Build history of the part. All positions in model axes, mm. Face numbers are marked on the shaded views. Round coordinates to 2 decimals unless told otherwise and drop trailing zeros. Loops run counter-clockwise (first coordinate to the right, second up) from the corner with the lowest first, then second, coordinate; pieces in that order, holes last. Notation, with made-up numbers: (55, 9.5) - (96, 9.5) arc R16 cw to (96, 34.5) - close; hole circle Ø2 at (1.5, 42.5). An arc over 180 degrees is marked (long way). Use a Markdown table: item, result.
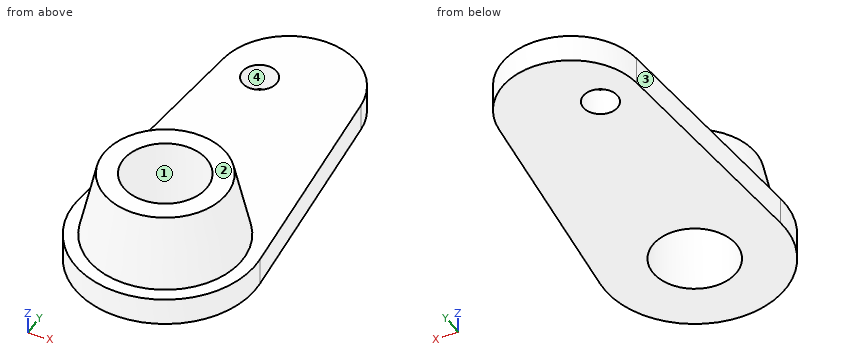
from build123d import *

# Parameters (mm, degrees)
F1_DEPTH = 12.7
F5_D     = 38.1
F7_D     = 15.748


with BuildPart() as f1:
    # F0 (on Top) → F1 (new body)
    with BuildSketch(Plane.XY):
        with BuildLine():
            Line((-31.362119, 109.072947), (-41.099551, 3.801645))
            ThreePointArc((-41.099551, 3.801645), (0, -41.275), (41.099551, 3.801645))
            Line((41.099551, 3.801645), (31.362119, 109.072947))
            ThreePointArc((31.362119, 109.072947), (0, 137.668), (-31.362119, 109.072947))
        make_face()
    extrude(amount=F1_DEPTH)

    # F2 (on Right) → F3 (revolve)
    with BuildSketch(Plane.YZ):
        Polygon((-27.94, 44.45), (-35.052, 12.7), (0, 12.7), (0, 44.45), align=None)
    revolve(axis=Axis((0, 0, 28.575), (0, 0, -1)))

    # F5 (through all)
    with Locations(Plane.XY.offset(44.45)):
        with Locations((0, 0)):
            Hole(F5_D / 2)

    # F7 (through all)
    with Locations(Plane.XY.offset(12.7)):
        with Locations((-12.939112, 105.38061)):
            Hole(F7_D / 2)


solid = f1.part
Q1. Probe line 1 (Y direction, x = -13.5, z = 9.5); line 2 (Z direction, x = 33, y = 58.5); line 3 (Y direction, x = 0, z = 30). List the from-to ranges inside material, lowest first.
Results found:
| item | result |
|---|---|
| line 1 | y = -39 to -13.44, 13.44 to 97.53, 113.23 to 134.63 |
| line 2 | z = 0 to 12.7 |
| line 3 | y = -31.18 to -19.05, 19.05 to 31.18 |
Q2. Cut at C-C, the plane z = 3. List the corners of the cut face in (x, y) (3 decimals).
Results found:
| item | result |
|---|---|
| outline | (-41.1, 3.802) arc R41.275 ccw (long way) to (41.1, 3.802) - (31.362, 109.073) arc R31.496 ccw to (-31.362, 109.073) - close; hole circle Ø15.748 at (-12.939, 105.381); hole circle Ø38.1 at (0, 0) |
Q3. Cut at D-D, the plane z = 37. List the corners of the cut face in (x, y), plus the area to 3 significant figures.
Results found:
| item | result |
|---|---|
| outline | circle Ø59.22 at (0, 0); hole circle Ø38.1 at (0, 0) |
| area | 1,610 mm2 |
Q4. Drop flat-ended pins along their axis: pin 1 (10 mm diameter, centred on x = -26.5, z = 5.5, fed in from -Y); pin 2 (2 mm diameter, centred on x = 11, z = 24, fed in from +Y); pin 3 (1.5 mm diameter, centred on x = 27, z = 38, fed in from +Y). Give the stop position or say it passes through.
Results found:
| item | result |
|---|---|
| pin 1 | stops at y = -35.23 |
| pin 2 | stops at y = 31.02 |
| pin 3 | stops at y = 13.25 |
Q5. Pull direction Y, two halves, no side cores. Call the marked faces 1, 2, 3 and 4: pulls with the +Y half, pulls with the -Y half, needs draft (parallel to the pull), parting line crosses it, or undercut.
Results found:
| item | result |
|---|---|
| face 1 | undercut |
| face 2 | needs draft |
| face 3 | pulls with the +Y half |
| face 4 | undercut |
Q6. Cut at A-A, the plane y = 0. List the corners of the cut face in (x, z) (3 decimals), plus the area to 3 significant figures.
Results found:
| item | result |
|---|---|
| outline | (-41.275, 0) - (-19.05, 0) - (-19.05, 44.45) - (-27.94, 44.45) - (-35.052, 12.7) - (-41.275, 12.7) - close; (19.05, 0) - (41.275, 0) - (41.275, 12.7) - (35.052, 12.7) - (27.94, 44.45) - (19.05, 44.45) - close |
| area | 1,350 mm2 |
Q7. Cut at B-B, the plane x = 0. List the corners of the cut face in (y, z) (3 decimals).
Results found:
| item | result |
|---|---|
| outline | (-41.275, 0) - (-19.05, 0) - (-19.05, 44.45) - (-27.94, 44.45) - (-35.052, 12.7) - (-41.275, 12.7) - close; (19.05, 0) - (137.668, 0) - (137.668, 12.7) - (35.052, 12.7) - (27.94, 44.45) - (19.05, 44.45) - close |
